from build123d import *

# Parameters (mm, degrees)
SKETCH1_W           = 128
SKETCH1_H           = 78.5
BOSS_EXTRUDE1_DEPTH = 11.2
SKETCH2_W           = 69
SKETCH2_H           = 49
CUT_EXTRUDE1_DEPTH  = 10
FILLET2_R           = 2
SKETCH3_R           = 1.2446
CUT_EXTRUDE2_DEPTH  = 10
CUT_EXTRUDE3_REACH  = 103.9
SKETCH5_W           = 26.3
SKETCH5_H           = 10
FILLET3_R           = 3.175


with BuildPart() as part:
    # Sketch1 → Boss-Extrude1 (new body)
    with BuildSketch(Plane.XY):
        Rectangle(SKETCH1_W, SKETCH1_H)
    extrude(amount=BOSS_EXTRUDE1_DEPTH)

    # Sketch2 → Cut-Extrude1 (cut)
    with BuildSketch(Plane.XY.offset(11.2)):
        Rectangle(SKETCH2_W, SKETCH2_H)
    extrude(amount=-CUT_EXTRUDE1_DEPTH, mode=Mode.SUBTRACT)

    # Fillet2
    fillet2_edges = [part.edges().sort_by_distance(p)[0] for p in [
        (34.5, 0, 11.2),
        (0, 24.5, 11.2),
        (-34.5, 0, 11.2),
        (0, -24.5, 11.2),
    ]]
    fillet(fillet2_edges, radius=FILLET2_R)

    # Sketch3 → Cut-Extrude2 (cut)
    with BuildSketch(Plane.XY.offset(11.2)):
        with Locations((0, 34)):
            Circle(SKETCH3_R)
        with Locations(Location((0, -34, 0), (0, 0, 180))):
            Circle(SKETCH3_R)
    extrude(amount=-CUT_EXTRUDE2_DEPTH, mode=Mode.SUBTRACT)

    # Sketch5 → Cut-Extrude3 (cut, up to next)
    with BuildSketch(Plane.XZ.offset(39.25), mode=Mode.PRIVATE) as cut_extrude3_sk1:
        with Locations((50.85, 5)):
            Rectangle(SKETCH5_W, SKETCH5_H)
    cut_extrude3_tool1 = extrude(cut_extrude3_sk1.sketch, amount=-CUT_EXTRUDE3_REACH, mode=Mode.PRIVATE) & part.part
    # Sketch5 → Cut-Extrude3 (cut, up to next)
    with BuildSketch(Plane.XZ.offset(39.25), mode=Mode.PRIVATE) as cut_extrude3_sk2:
        with Locations((-50.85, 5)):
            Rectangle(SKETCH5_W, SKETCH5_H)
    cut_extrude3_tool2 = extrude(cut_extrude3_sk2.sketch, amount=-CUT_EXTRUDE3_REACH, mode=Mode.PRIVATE) & part.part
    add(cut_extrude3_tool1.solids().sort_by_distance((50.85, -39.25, 5))[0], mode=Mode.SUBTRACT)
    add(cut_extrude3_tool2.solids().sort_by_distance((-50.85, -39.25, 5))[0], mode=Mode.SUBTRACT)

    # Fillet3
    fillet3_edges = [part.edges().sort_by_distance(p)[0] for p in [
        (0, -39.25, 0),
        (0, 39.25, 0),
        (37.7, 0, 0),
        (-37.7, 0, 0),
        (64, -39.25, 10.6),
        (-64, -39.25, 10.6),
        (-64, 39.25, 10.6),
        (64, 39.25, 10.6),
    ]]
    fillet(fillet3_edges, radius=FILLET3_R)


solid = part.part
Read the model definition and answer for the solid it produces. Units are mm, in the model's axes. A direction names the side the tool comes from. Round coordinates to 2 decimals unless told otherwise and drop trailing zeros. Order: outer loops, then holes, each group sorted by start corner. A loop starts at its lowest first (then second) coordinate and runs counter-clockwise, first axis right, second up. Notation, with made-up numbers: (34.5, -19) - (61.5, -19) arc R9 ccw to (61.5, -13) - close; hole circle Ø1 at (86.25, 52). An arc over 180 degrees is marked (long way). Use one line per item in the form item = value. Start each with the question number.
(1) Find the intervals of material crossed by line 1 along Y through (x, z) = (0, 8.5); line 2 along X through (y, z) = (-34, 6.25); line 3 along Y through (x, z) = (-34, 6.5), in increasing order. Write a range as from..to.
(2) Determine the mould class of faces 1 (the face through (-34.5, 0, 5)), 2 (the face through (-1, -39.25, 7)), 3 (the face through (37.7, -1, 7)) for opening direction X: +X half, -X half, draft (parallel to the pull), parting line (faces both ways), or undercut.
(3) The part is cut by section A-A (y = -4.5). Give the vertices of the cut face in (x, z) (3 decimals).
(4) Flat-ended cylindrical pins translate along their axes: pin 1 Ø6.5 at (y, z) = (2.5, 3.5) entering from -X; pin 2 Ø21 at (x, y) = (-55, -6) entering from -Z; pin 3 Ø24.5 at (x, y) = (8, 5.5) entering from +Z; pin 4 Ø6 at (x, z) = (-48, 4.5) entering from -Y. Find the tip coordinate at first contact, or state that the pin passes through.
(5) The part is cut by section C-C (x = 27.5). Give the vertices of the cut face in (y, z) (3 decimals).
(6) The part is cut by section B-B (z = 7.25). Give the vertices of the cut face in (x, y).
(7) For faces 4 (the face through (-63.09, -38.3, 10.61)), 5 (the face through (-37.7, -1, 7)), 6 (the face through (0, 24.5, 5)), determine the directions among +Z, -Z, +X, -X, +Y, -Y from which every point of the face is accessible in a straight line to the end or side of a thin tool.
(8) The part is cut by section D-D (y = 34). Give the vertices of the cut face in (x, z) (3 decimals), then the cut area to 3 significant figures.
Checked values:
q1.line_1 = -39.25..-35.24, -32.76..-24.5, 24.5..32.76, 35.24..39.25
q1.line_2 = -37.7..-1.24, 1.24..37.7
q1.line_3 = -39.25..-24.5, 24.5..39.25
q2.face_1 = undercut
q2.face_2 = draft
q2.face_3 = +X half
q3.outline = (-64, 10) - (-37.7, 10) - (-37.7, 3.175) arc R3.175 ccw to (-34.525, 0) - (34.525, 0) arc R3.175 ccw to (37.7, 3.175) - (37.7, 10) - (64, 10) - (64, 11.2) - (36.5, 11.2) arc R2 ccw to (34.5, 9.2) - (34.5, 1.2) - (-34.5, 1.2) - (-34.5, 9.2) arc R2 ccw to (-36.5, 11.2) - (-64, 11.2) - close
q4.pin_1 = -37.7
q4.pin_2 = 10
q4.pin_3 = 1.2
q4.pin_4 = through
q5.outline = (-39.25, 3.175) arc R3.175 ccw to (-36.075, 0) - (36.075, 0) arc R3.175 ccw to (39.25, 3.175) - (39.25, 11.2) - (26.5, 11.2) arc R2 ccw to (24.5, 9.2) - (24.5, 1.2) - (-24.5, 1.2) - (-24.5, 9.2) arc R2 ccw to (-26.5, 11.2) - (-39.25, 11.2) - close
q6.outline = (-37.7, -39.25) - (37.7, -39.25) - (37.7, 39.25) - (-37.7, 39.25) - close; hole (-34.5, -24.5) - (34.5, -24.5) - (34.5, 24.5) - (-34.5, 24.5) - close; hole circle Ø2.49 at (0, -34); hole circle Ø2.49 at (0, 34)
q7.face_4 = +Z, -Z, -X, -Y
q7.face_5 = -Z, -X, +Y, -Y
q7.face_6 = +Z
q8.outline = (-64, 10) - (-37.7, 10) - (-37.7, 3.175) arc R3.175 ccw to (-34.525, 0) - (34.525, 0) arc R3.175 ccw to (37.7, 3.175) - (37.7, 10) - (64, 10) - (64, 11.2) - (1.245, 11.2) - (1.245, 1.2) - (-1.245, 1.2) - (-1.245, 11.2) - (-64, 11.2) - close
q8.area = 878 mm^2
